```python
from build123d import *

# Parameters (mm, degrees)
F0_R     = 1.5
F1_DEPTH = 6
F2_DEPTH = 240
F4_R     = 2


with BuildPart() as f1:
    # F0 (on Top) → F1 (new body)
    with BuildSketch(Plane.XY):
        Polygon((-4, 2.3094010768), (-4, -2.3094010768), (0, -4.6188021535), (4, -2.3094010768), (4, 2.3094010768), (0, 4.6188021535), align=None)
        Circle(F0_R, mode=Mode.SUBTRACT)
    extrude(amount=F1_DEPTH)

    # F2 (add): a face of the model
    f2_faces = [f1.faces().sort_by_distance(p)[0] for p in [
        (4, 0, 3),
    ]]
    extrude(f2_faces, amount=F2_DEPTH)

    # F3: F1 across face


with BuildPart() as f1_1:
    add(f1.part)
    add(f1.part.mirror(Plane(origin=(244, 0, 3), x_dir=(0, 1, 0), z_dir=(1, 0, 0))))

    # F4
    f4_edges = [f1_1.edges().sort_by_distance(p)[0] for p in [
        (244, -2.309401, 6),
        (244, 2.309401, 6),
        (244, -2.309401, 0),
        (244, 2.309401, 0),
    ]]
    fillet(f4_edges, radius=F4_R)


solid = f1_1.part
```
Could you check a few things on this model? Use its own coordinates, in mm. Round coordinates to 2 decimals unless told otherwise and drop trailing zeros. Loops run counter-clockwise (first coordinate to the right, second up) from the corner with the lowest first, then second, coordinate; pieces in that order, holes last. Notation, with made-up numbers: (63.5, -27) - (69.5, -27) arc R25 ccw to (69.5, 8) - close; hole circle Ø9 at (5, 25). An arc over 180 degrees is marked (long way). Answer in a Markdown table with one row per item. Add a question column.
(1) If we section it at A-A (x = 393.5): Please give me the cut outline in (y, z).
(2) I need wall thicknesses on line 1 along X through (y, z) = (0.25, 3.1); line 2 along Y through (x, z) = (0, 2); line 3 along Y through (x, z) = (70.5, 3.4). Which ranges of each line are inside material? Lowest first, please.
(3) If we section it at B-B (z = 4.95): Please give me the cut outline in (x, y), plus the area to 3 significant figures.
(4) I'm going to push flat-ended pins straight in: pin 1 (1.6 mm diameter, centred on x = 141.5, z = 3, fed in from +Y); pin 2 (1.5 mm diameter, centred on x = 132.5, z = 2.5, fed in from -Y); pin 3 (2 mm diameter, centred on x = 154, y = 2.5, fed in from +Z). Where does each tip first touch, or does it pass through?
Model answer:
| question | item | result |
|---|---|---|
| 1 | outline | (-2.31, 2) arc R2 ccw to (-0.31, 0) - (0.31, 0) arc R2 ccw to (2.31, 2) - (2.31, 4) arc R2 ccw to (0.31, 6) - (-0.31, 6) arc R2 ccw to (-2.31, 4) - close |
| 2 | line 1 | x = -4 to -1.48, 1.48 to 486.52, 489.48 to 492 |
| 2 | line 2 | y = -4.62 to -1.5, 1.5 to 4.62 |
| 2 | line 3 | y = -2.31 to 2.31 |
| 3 | outline | (-4, -2.31) - (0, -4.62) - (4.42, -2.07) - (483.58, -2.07) - (488, -4.62) - (492, -2.31) - (492, 2.31) - (488, 4.62) - (483.58, 2.07) - (4.42, 2.07) - (0, 4.62) - (-4, 2.31) - close; hole circle Ø3 at (0, 0); hole circle Ø3 at (488, 0) |
| 3 | area | 2,080 mm² |
| 4 | pin 1 | stops at y = 2.31 |
| 4 | pin 2 | stops at y = -2.31 |
| 4 | pin 3 | stops at z = 5.61 |
